For this review, use the dimensioned drawing (mm, ordinates from the lowest corner) and the shaded views. A direction names the side the tool comes from. Give positions to 0.01 mm unless a question says otherwise; leave off trailing zeros. Loops run counter-clockwise (first coordinate to the right, second up) from the corner with the lowest first, then second, coordinate; pieces in that order, holes last. Notation, with made-up numbers: (45.5, -17.75) -> (103.5, -17.75) arc R34 ccw to (103.5, 15.25) -> close; hole circle Ø2 at (55, 73.5). An arc over 180 degrees is marked (long way). Write each question's results on one line, items separated by ' | '. Start each with the question number.
Q1. Insertion check: pin 1 Ø1.5 at (x, y) = (19.5, 6) entering from +Z; pin 2 Ø10 at (x, z) = (8.5, 18.5) entering from +Y. Each pin has a flat end and moves straight along its axis. Give the tip position at first contact, or say it passes through.
Q2. We need section D-D (x = 15.25). Write out the cut boundary in (y, z).
Q3. Wall thickness on L1, parallel to X at y = 8, z = 10.25; L2, parallel to Z at x = 12.5, y = 1.05; L3, parallel to Y at x = 12.5, z = 2.2: over which ranges is each line inside the solid? List them lowest first. Write a range as [from, to].
Q4. We need section C-C (z = 10). Write out the cut boundary in (x, y).
Q5. We need section A-A (x = 12.5). Write out the cut boundary in (y, z).
Q6. We need section B-B (y = 15). Write out the cut boundary in (x, z), plus the area to 3 significant figures.
Q7. Machinability: for the marked faces 1 and 2, which of the approach directions +Z, -Z, +X, -X, +Y, -Y give a long, thin tool a straight path to every point of the face, cutting with its end or side? Answer none if there is none.
Q8. Mouldability with a two-part tool opening along X and no side actions: class the marked faces 3, 4 and 5 as released by +X, released by -X, zero draft, split by the parting line, or undercut.
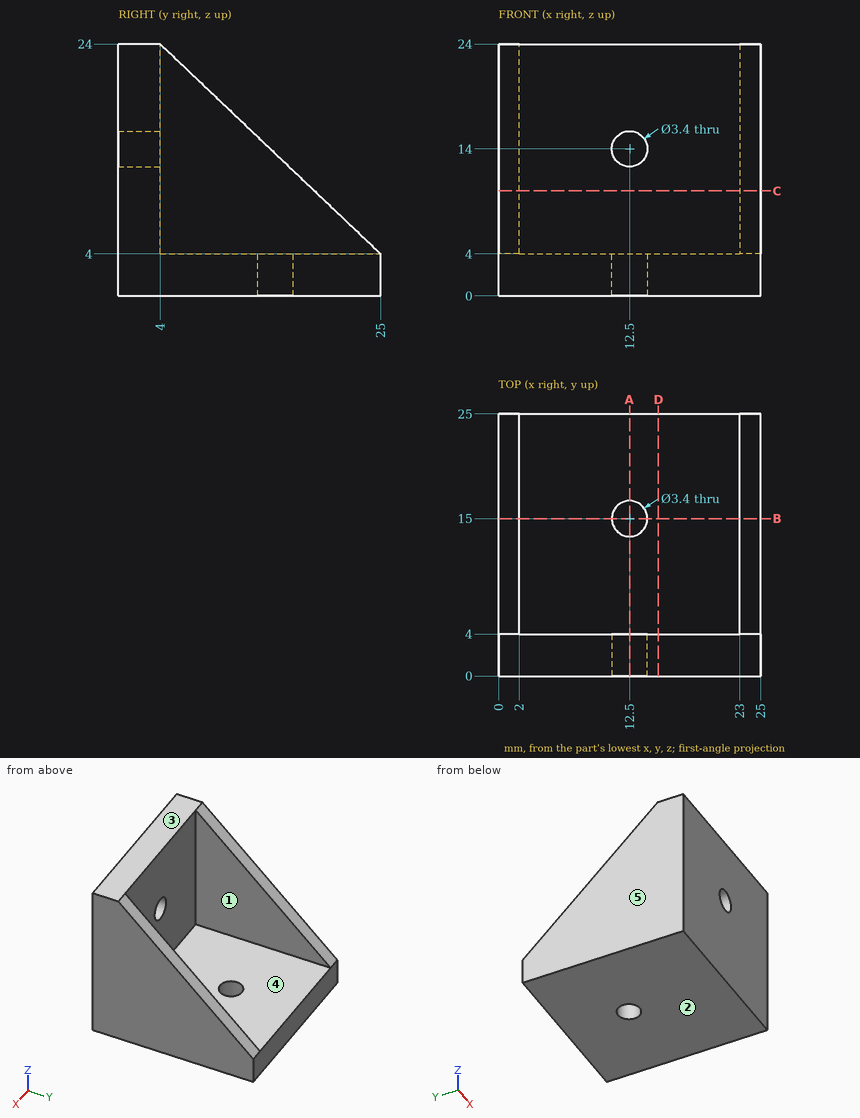
Output:
1) pin 1: z = 4 | pin 2: y = 4
2) outline: (0, 0) -> (25, 0) -> (25, 4) -> (4, 4) -> (4, 24) -> (0, 24) -> close
3) L1: [0, 2], [23, 25] | L2: [0, 12.3], [15.7, 24] | L3: [0, 13.3], [16.7, 25]
4) outline: (0, 0) -> (25, 0) -> (25, 18.7) -> (23, 18.7) -> (23, 4) -> (2, 4) -> (2, 18.7) -> (0, 18.7) -> close
5) outline: (0, 0) -> (13.3, 0) -> (13.3, 4) -> (4, 4) -> (4, 12.3) -> (0, 12.3) -> close; (0, 15.7) -> (4, 15.7) -> (4, 24) -> (0, 24) -> close; (16.7, 0) -> (25, 0) -> (25, 4) -> (16.7, 4) -> close
6) outline: (0, 0) -> (10.8, 0) -> (10.8, 4) -> (2, 4) -> (2, 13.52) -> (0, 13.52) -> close; (14.2, 0) -> (25, 0) -> (25, 13.52) -> (23, 13.52) -> (23, 4) -> (14.2, 4) -> close | area: 124 mm2
7) face 1: +Z, +Y | face 2: -Z, +X, -X, +Y, -Y
8) face 3: zero draft | face 4: undercut | face 5: released by -X
